Source: CAD feature listing. Evaluate the final solid. Frame: model axes, mm. A direction names the side the tool comes from. Round coordinates to 2 decimals unless told otherwise and drop trailing zeros. Order: outer loops, then holes, each group sorted by start corner. A loop starts at its lowest first (then second) coordinate and runs counter-clockwise, first axis right, second up. Notation, with made-up numbers: (18.5, 56) -> (35.5, 56) arc R19 cw to (35.5, 77) -> close; hole circle Ø8 at (12, 53). An arc over 180 degrees is marked (long way). Answer as CSV lines item,"result".
from build123d import *

# Parameters (mm, degrees)
F2_DEPTH = 200
F3_W     = 30
F3_H     = 100
F4_DEPTH = 500
F6_R     = 15
F7_R     = 5
F8_W     = 101.1056527495
F8_H     = 22.9697218165
F9_DEPTH = 200
F10_R    = 5


with BuildPart() as f2:
    # F0 (on Front) → F2 (new body)
    with BuildSketch(Plane.XZ):
        with BuildLine():
            Line((-127.5536519289, -36.5021181107), (-127.5536519289, 43.4978818893))
            Line((-127.5536519289, 43.4978818893), (-132.5536519289, 43.4978818893))
            Line((-132.5536519289, 43.4978818893), (-132.5536519289, -36.5021181107))
            ThreePointArc((-132.5536519289, -36.5021181107), (-125.2313214586, -54.1797876403), (-107.5536519289, -61.5021181107))
            Line((-107.5536519289, -61.5021181107), (102.4463480711, -61.5021181107))
            ThreePointArc((102.4463480711, -61.5021181107), (120.1240176008, -54.1797876403), (127.4463480711, -36.5021181107))
            Line((127.4463480711, -36.5021181107), (127.4463480711, 43.4978818893))
            Line((127.4463480711, 43.4978818893), (122.4463480711, 43.4978818893))
            Line((122.4463480711, 43.4978818893), (122.4463480711, -36.5021181107))
            ThreePointArc((122.4463480711, -36.5021181107), (116.5884836948, -50.6442537344), (102.4463480711, -56.5021181107))
            Line((102.4463480711, -56.5021181107), (-107.5536519289, -56.5021181107))
            ThreePointArc((-107.5536519289, -56.5021181107), (-121.6957875526, -50.6442537344), (-127.5536519289, -36.5021181107))
        make_face()
    extrude(amount=F2_DEPTH)


with BuildPart() as f4:
    # F3 (on offset) → F4 (new body)
    with BuildSketch(Plane.YZ.offset(200)):
        with Locations((-145, -29.9103426556)):
            Rectangle(F3_W, F3_H)
    extrude(amount=-F4_DEPTH)


with BuildPart() as f4b:
    # F3 (on offset) → F4, piece 2 (new body)
    with BuildSketch(Plane.YZ.offset(200)):
        with Locations((-35, -29.9103426556)):
            Rectangle(F3_W, F3_H)
    extrude(amount=-F4_DEPTH)


with BuildPart() as f2_1:
    add(f2.part)

    # F5: cut F4, F4b
    add(f4.part, mode=Mode.SUBTRACT)
    add(f4b.part, mode=Mode.SUBTRACT)

    # F6
    f6_edges = [f2_1.edges().sort_by_distance(p)[0] for p in [
        (-130.053652, -200, 43.497882),
        (-130.053652, 0, 43.497882),
        (124.946348, -200, 43.497882),
        (124.946348, 0, 43.497882),
    ]]
    fillet(f6_edges, radius=F6_R)

    # F7
    f7_edges = [f2_1.edges().sort_by_distance(p)[0] for p in [
        (124.946348, -20, 20.089657),
        (124.946348, -50, 20.089657),
    ]]
    fillet(f7_edges, radius=F7_R)

    # F8 (on offset) → F9 (cut)
    with BuildSketch(Plane.YZ.offset(200)):
        with Locations((-91.6927345097, -2.6946733706)):
            Rectangle(F8_W, F8_H)
    extrude(amount=-F9_DEPTH, mode=Mode.SUBTRACT)

    # F10
    f10_edges = [f2_1.edges().sort_by_distance(p)[0] for p in [
        (124.946348, -50, -14.179534),
        (124.946348, -50, 8.790188),
        (124.946348, -130, 8.790188),
        (124.946348, -130, -14.179534),
        (124.946348, -130, 20.089657),
        (124.946348, -160, 20.089657),
    ]]
    fillet(f10_edges, radius=F10_R)


solid = f2_1.part
1. Section query A-A on z = -22. Return loops of the section in (x, y).
Results below:
outline,"(-132.55, -200) -> (-127.55, -200) -> (-127.55, -160) -> (-132.55, -160) -> close; (-132.55, -130) -> (-127.55, -130) -> (-127.55, -50) -> (-132.55, -50) -> close; (-132.55, -20) -> (-127.55, -20) -> (-127.55, 0) -> (-132.55, 0) -> close; (122.45, -200) -> (127.45, -200) -> (127.45, -160) -> (122.45, -160) -> close; (122.45, -130) -> (127.45, -130) -> (127.45, -50) -> (122.45, -50) -> close; (122.45, -20) -> (127.45, -20) -> (127.45, 0) -> (122.45, 0) -> close"
2. Reachability of faces 4 (the flat face through (-127.554, -99, 3)), 5 (the cylindrical face through (119.9, -179.7, -54.4)) from +Z, -Z, +X, -X, +Y, -Y: full face, straight path, thin tool, end or side. Return the list, or none.
Results below:
face 4,"+Z, +Y, -Y"
face 5,"-Z, +X, +Y, -Y"
3. Pin query (flat end, axial travel): pin 1 (5.5 mm diameter, centred on x = -130.5, y = -33, fed in from -Z); pin 2 (10 mm diameter, centred on x = 78, z = -50.5, fed in from +Y); pin 3 (5.5 mm diameter, centred on x = 126, y = -77, fed in from -Z); pin 4 (24 mm diameter, centred on x = -18, y = -81, fed in from +Z). Return the tip coordinate at first contact, or that it passes through.
Results below:
pin 1,"z = 20.09"
pin 2,"through"
pin 3,"z = -50.37"
pin 4,"z = -56.5"
4. Section query B-B on x = 65.5. Return loops of the section in (y, z), and give its area (3 significant figures).
Results below:
outline,"(-200, -61.5) -> (-160, -61.5) -> (-160, -56.5) -> (-200, -56.5) -> close; (-130, -61.5) -> (-50, -61.5) -> (-50, -56.5) -> (-130, -56.5) -> close; (-20, -61.5) -> (0, -61.5) -> (0, -56.5) -> (-20, -56.5) -> close"
area,"700 mm2"
5. Section query D-D on y = -74. Return loops of the section in (x, z).
Results below:
outline,"(-132.55, -36.5) arc R25 ccw to (-107.55, -61.5) -> (102.45, -61.5) arc R25 ccw to (127.45, -36.5) -> (127.45, -14.18) -> (122.45, -14.18) -> (122.45, -36.5) arc R20 cw to (102.45, -56.5) -> (-107.55, -56.5) arc R20 cw to (-127.55, -36.5) -> (-127.55, 43.5) -> (-132.55, 43.5) -> close; (122.45, 8.79) -> (127.45, 8.79) -> (127.45, 43.5) -> (122.45, 43.5) -> close"
6. Section query C-C on z = 6. Return loops of the section in (x, y), and give its area (3 significant figures).
Results below:
outline,"(-132.55, -200) -> (-127.55, -200) -> (-127.55, -160) -> (-132.55, -160) -> close; (-132.55, -130) -> (-127.55, -130) -> (-127.55, -50) -> (-132.55, -50) -> close; (-132.55, -20) -> (-127.55, -20) -> (-127.55, 0) -> (-132.55, 0) -> close; (122.45, -200) -> (127.45, -200) -> (127.45, -160) -> (122.45, -160) -> close; (122.45, -20) -> (127.45, -20) -> (127.45, 0) -> (122.45, 0) -> close"
area,"1,000 mm2"
7. Mould query, pull axis X, two halves, no side actions, for faces 1 (the flat face through (-132.554, -99, 4)), 2 (the flat face through (122.446, -89, -25)), 3 (the cylindrical face through (119.9, -9.9, -54.4)). Classes: released by +X, released by -X, zero draft, split by the parting line, or undercut.
Results below:
face 1,"released by -X"
face 2,"undercut"
face 3,"released by +X"
8. Line query: L1, parallel to X at y = -184, z = -16; L2, parallel to Z at x = 59.5, y = -74; L3, parallel to Z at x = 107, y = -101. Output: solid intervals per line, ascending. Write a range as [from, to].
Results below:
L1,"[-132.55, -127.55], [122.45, 127.45]"
L2,"[-61.5, -56.5]"
L3,"[-61.08, -55.98]"
